Here's the drawing with two shaded views (mm, measured from the low corner). I have some questions. Round coordinates to 2 decimals unless told otherwise and drop trailing zeros. Write each loop counter-clockwise with the first axis right and the second up, starting at its lowest first coordinate (ties: lowest second). Pieces come first, ordered by that corner, then holes. Notation, with made-up numbers: M -28.5,52 L 22.5,52 A17 cw 22.5,64 Z; hole C 85,75.5 d3. An arc over 180 degrees is marked long. Answer as a JSON object with one key per item and string values. Group by question number.
1) Suppose I cut it at B-B, the plane x = 348.45. Write out the boundary of the cut face in (y, z).
2) Suppose I cut it at A-A, the plane y = 44.45. Write out the boundary of the cut face in (x, z), and give its area (3 significant figures).
3) Please list where these lines run through material, in increasing order: L1, parallel to Y at x = 348.45, z = 6.5; L2, parallel to X at y = 47, z = 2.5. Write a range as [from, to].
4) I'm going to push a flat-ended pin straight in: pin 1 Ø1.5 at (x, z) = (506, 16.5) entering from -Y. Where does the tip first touch, or does it pass through?
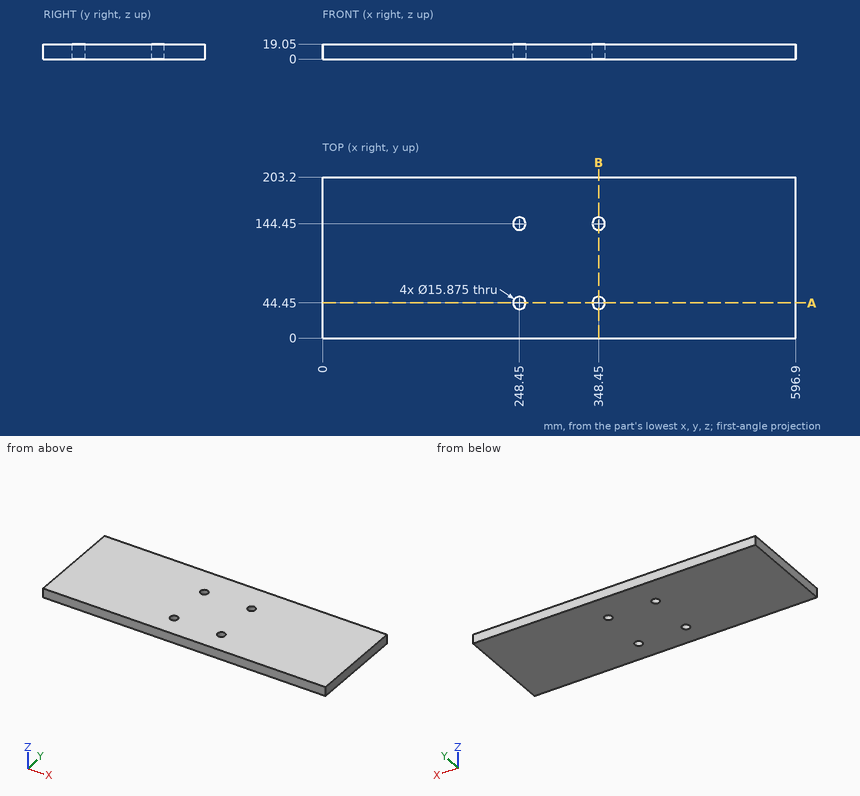
Results:
{
 "1": {"outline": "M 0,0 L 36.51,0 L 36.51,19.05 L 0,19.05 Z; M 52.39,0 L 136.51,0 L 136.51,19.05 L 52.39,19.05 Z; M 152.39,0 L 203.2,0 L 203.2,19.05 L 152.39,19.05 Z"},
 "2": {"outline": "M 0,0 L 240.51,0 L 240.51,19.05 L 0,19.05 Z; M 256.39,0 L 340.51,0 L 340.51,19.05 L 256.39,19.05 Z; M 356.39,0 L 596.9,0 L 596.9,19.05 L 356.39,19.05 Z", "area": "10,800 mm^2"},
 "3": {"L1": "[0, 36.51], [52.39, 136.51], [152.39, 203.2]", "L2": "[0, 240.93], [255.97, 340.93], [355.97, 596.9]"},
 "4": {"pin 1": "y = 0"}
}
